Autodesk Inventor part; units mm, degrees
ref_plane "YZ Plane" through (0, 0, 0) normal (1, 0, 0) x (0, 1, 0)
ref_plane "XZ Plane" through (0, 0, 0) normal (0, 1, 0) x (-1, 0, 0)
ref_plane "XY Plane" through (0, 0, 0) normal (0, 0, 1) x (1, 0, 0)
sketch "Sketch1" plane through (0, 0, 0) normal (0, 1, 0) x (-1, 0, 0)
  line L0 (0, 0) -> (22, 0)
  line L1 (22, 0) -> (22, -20)
  line L2 (22, -20) -> (0, -20)
  line L3 (0, -20) -> (0, 0)
  dimension "d2" = 20
  dimension "d3" = 22
extrude "Extrusion1" add sketch "Sketch1" along normal blind 3
sketch "Sketch3" plane through (0, 3, 0) normal (0, 1, 0) x (1, 0, 0)
  line L0 (0, 0) -> (-3, 0)
  line L1 (-3, 0) -> (-3, 20)
  line L2 (-3, 20) -> (0, 20)
  line L3 (0, 20) -> (0, 0)
  line L4 (-22, 0) -> (0, 0)
  line L5 (0, 20) -> (-22, 20)
  line L6 (-11.5, 0) -> (-8.5, 0)
  line L7 (-8.5, 0) -> (-8.5, 20)
  line L8 (-8.5, 20) -> (-11.5, 20)
  line L9 (-11.5, 20) -> (-11.5, 0)
  dimension "d8" = 3
  dimension "d25" = 3
  dimension "d26" = 5.5
extrude "Extrusion2" add sketch "Sketch3" along normal blind 15 contours L0 L1 L2 L3 | L4 L9 L5 L7
sketch "Sketch4" plane through (0, 0, 0) normal (1, 0, 0) x (0, 0, -1)
  line L0 (0, 3) -> (0, 18)
  line L1 (0, 13) -> (20.043, 13)
  line L2 (0, 18) -> (20, 18)
  circle A0 centre (5, 13) radius 2.75
  circle A1 centre (15, 13) radius 2.75
  line L3 (20, 0) -> (20, 18)
  point P0 (0, 0)
  dimension "d11" = 5
  dimension "d12" = 10
  dimension "d13" = 5.5
  dimension "d14" = 5.5
  dimension "d15" = 5
extrude "Extrusion3" cut sketch "Sketch4" against normal blind 29.25 contours A0 L1 | L1 A0 | A1 L1 | L1 A1
sketch "Sketch5" plane through (0, 0, 0) normal (0, -1, 0) x (1, 0, 0)
  line L0 (-22, 0) -> (0, 0)
  line L1 (-16, 0) -> (-16, -20)
  line L2 (0, -20) -> (-22, -20)
  line L3 (-22, -20) -> (-22, 0)
  circle A0 centre (-16, -10) radius 4.25
  dimension "d18" = 6
  dimension "d19" = 8.5
  dimension "d27" = 10
extrude "Extrusion4" cut sketch "Sketch5" against normal blind 1 contours A0 L1 | L1 A0
sketch "Sketch6" plane through (-16, 1, -10) normal (0, -1, 0) x (1, 0, 0)
  circle A0 centre (0, 0) radius 2.75
  point P0 (16, 10)
  dimension "d22" = 5.5
extrude "Extrusion5" cut sketch "Sketch6" against normal blind 9
fillet "Fillet1" radius 6 2 edges at (-22, 1.5, -20) (-22, 1.5, 0)
properties part number "XY_Zfixer" material "Thermoplastic Resin"
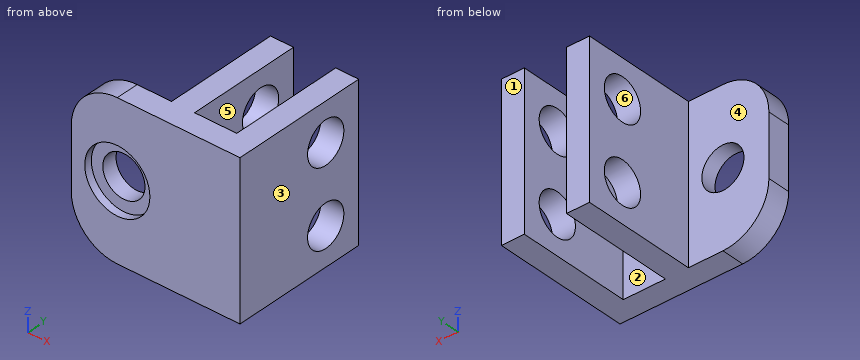
The model under review builds one solid part; all positions refer to its coordinate system, in mm. Face numbers are marked on the shaded views. A direction names the side the tool comes from. Round coordinates to 2 decimals unless told otherwise and drop trailing zeros. Write each loop counter-clockwise with the first axis right and the second up, starting at its lowest first coordinate (ties: lowest second). Pieces come first, ordered by that corner, then holes. Notation, with made-up numbers: M -15,37 L 32,37 A23 cw 32,57 Z; hole C -23,60 d1. An arc over 180 degrees is marked long. Use CSV: the item, a comma, the result in double quotes. Start each with the question number.
(1) Tool access review of the marked faces 4, 5 and 6: name each direction out of +Z, -Z, +X, -X, +Y, -Y from which nothing blocks a thin tool from reaching the whole face with its end or side.
(2) We need section A-A, the plane z = -10. State the section outline as (x, y) points, then the cut area to 4 significant figures.
(3) We need section B-B, the plane y = 8.5. State the section outline as (x, z) points.
(4) We need section C-C, the plane x = -1.75. State the section outline as (y, z) points, then the cut area to 3 significant figures.
(5) For line 1 along Z through (x, y) = (-2, 13); line 2 along Y through (x, z) = (-9.65, -5); line 3 along X through (y, z) = (5.5, -17.5), list the stretches that pass through material, from the lowest coordinate up.
(6) The part is to be moulded in two halves that separate along X. For the marked faces 1, 2 and 3, say which applies: +X half, -X half, draft (parallel to the pull), parting line (faces both ways), or undercut.
(7) Clearance check with flat-ended pins moving along their axes: P1, Ø5, axis at x = -14.5, z = -5.5, coming from the +Y side; P2, Ø4, axis at x = -16.5, z = -8, coming from the -Y side; P3, Ø5, axis at y = 11.5, z = -11.5, coming from the -X side. State where each tip first meets the part, or that it passes through.
(8) We need section D-D, the plane y = 13. State the section outline as (x, z) points.
Findings:
1,face 4,"+Z, -Z, -X, +Y"
1,face 5,"+Z, -Z, +Y"
1,face 6,"+X, -X"
2,outline,"M -22,0 L -20.25,0 L -20.25,1 L -18.75,1 L -18.75,3 L -22,3 Z; M -13.25,1 L -11.75,1 L -11.75,0 L 0,0 L 0,18 L -3,18 L -3,3 L -8.5,3 L -8.5,18 L -11.5,18 L -11.5,3 L -13.25,3 Z"
2,area,"136.5 mm^2"
3,outline,"M -11.5,-20 L -8.5,-20 L -8.5,0 L -11.5,0 Z; M -3,-20 L 0,-20 L 0,0 L -3,0 Z"
4,outline,"M 0,-20 L 18,-20 L 18,0 L 0,0 Z; hole C 13,-15 d5.5; hole C 13,-5 d5.5"
4,area,"312 mm^2"
5,line 1,"-20 to -17.75, -12.25 to -7.75, -2.25 to 0"
5,line 2,"0 to 10.25, 15.75 to 18"
5,line 3,"-11.5 to -8.5, -3 to 0"
6,face 1,"draft"
6,face 2,"undercut"
6,face 3,"+X half"
7,P1,"y = 3"
7,P2,"y = 1"
7,P3,"x = -11.5"
8,outline,"M -11.5,-20 L -8.5,-20 L -8.5,-17.75 L -11.5,-17.75 Z; M -11.5,-12.25 L -8.5,-12.25 L -8.5,-7.75 L -11.5,-7.75 Z; M -11.5,-2.25 L -8.5,-2.25 L -8.5,0 L -11.5,0 Z; M -3,-20 L 0,-20 L 0,-17.75 L -3,-17.75 Z; M -3,-12.25 L 0,-12.25 L 0,-7.75 L -3,-7.75 Z; M -3,-2.25 L 0,-2.25 L 0,0 L -3,0 Z"
